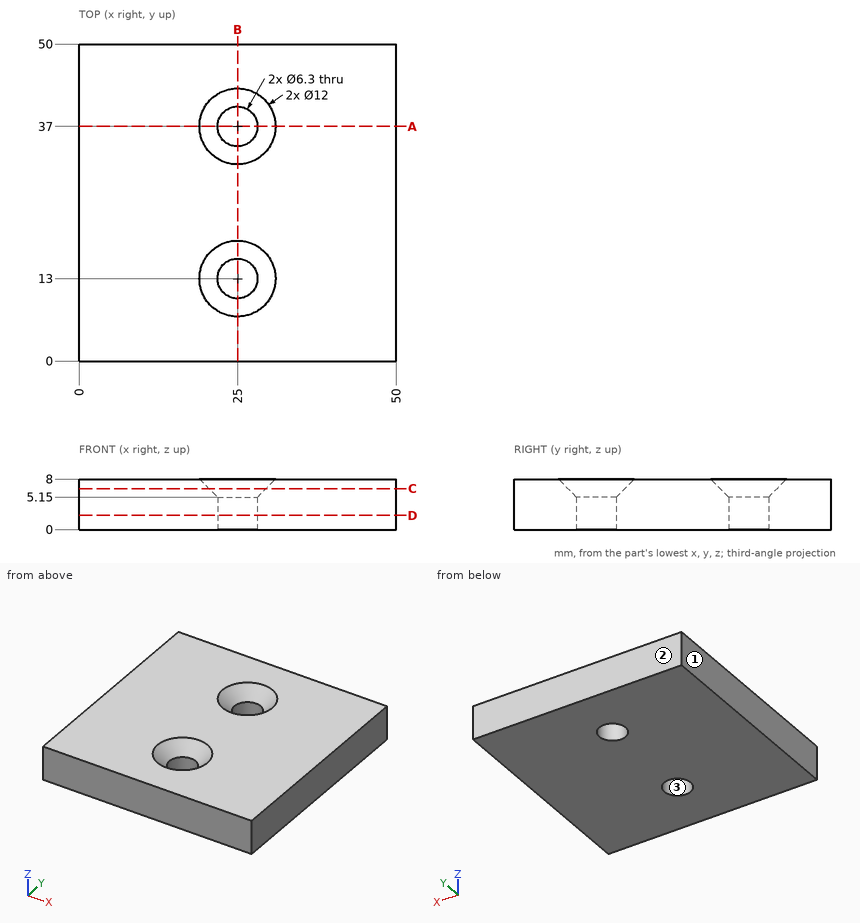
Can you work these out from the drawing? Everything is in mm from the part's minimum corner. Round coordinates to 2 decimals unless told otherwise and drop trailing zeros. Loops run counter-clockwise (first coordinate to the right, second up) from the corner with the lowest first, then second, coordinate; pieces in that order, holes last. Notation, with made-up numbers: M 22.5,27 L 72.5,27 A15 ccw 72.5,42 Z; hole C 24,60 d1. An arc over 180 degrees is marked long. Answer in a Markdown table with one row per item.
1. If we section it at B-B, the plane x = 25: Please give me the cut outline in (y, z), plus the area to 3 significant figures.
Established:
| item | result |
|---|---|
| outline | M 0,0 L 9.85,0 L 9.85,5.15 L 7,8 L 0,8 Z; M 16.15,0 L 33.85,0 L 33.85,5.15 L 31,8 L 19,8 L 16.15,5.15 Z; M 40.15,0 L 50,0 L 50,8 L 43,8 L 40.15,5.15 Z |
| area | 283 mm² |
2. Please list where these lines run through material, in increasing order: line 1 (Y direction, x = 25, z = 3); line 2 (X direction, y = 37, z = 1.2); line 3 (X direction, y = 38.5, z = 5.5). Write a range as from..to.
Established:
| item | result |
|---|---|
| line 1 | 0..9.85, 16.15..33.85, 40.15..50 |
| line 2 | 0..21.85, 28.15..50 |
| line 3 | 0..21.84, 28.16..50 |
3. Thinking about a two-plate mould opening in Y: for the marked faces 1, 2 and 3, which applies, pulls with the +Y half, pulls with the -Y half, needs draft (parallel to the pull), parting line crosses it, or undercut?
Established:
| item | result |
|---|---|
| face 1 | needs draft |
| face 2 | pulls with the +Y half |
| face 3 | undercut |
4. If we section it at C-C, the plane z = 6.5: Please give me the cut outline in (x, y), plus the area to 3 significant figures.
Established:
| item | result |
|---|---|
| outline | M 0,0 L 50,0 L 50,50 L 0,50 Z; hole C 25,13 d9; hole C 25,37 d9 |
| area | 2,370 mm² |
5. If we section it at A-A, the plane y = 37: Please give me the cut outline in (x, z), plus the area to 3 significant figures.
Established:
| item | result |
|---|---|
| outline | M 0,0 L 21.85,0 L 21.85,5.15 L 19,8 L 0,8 Z; M 28.15,0 L 50,0 L 50,8 L 31,8 L 28.15,5.15 Z |
| area | 341 mm² |
6. If we section it at D-D, the plane z = 2.25: Please give me the cut outline in (x, y), plus the area to 3 significant figures.
Established:
| item | result |
|---|---|
| outline | M 0,0 L 50,0 L 50,50 L 0,50 Z; hole C 25,13 d6.3; hole C 25,37 d6.3 |
| area | 2,440 mm² |
